from build123d import *

# Parameters (mm, degrees)
F0_W           = 15
F0_H           = 50
F1_DEPTH       = 20
F3_D           = 5.5
F3_CBORE_D     = 9.5
F3_CBORE_DEPTH = 5.4
F4_SIZE        = 1


with BuildPart() as f1:
    # F0 (on Top) → F1 (new body)
    with BuildSketch(Plane.XY):
        with Locations((7.5, 25)):
            Rectangle(F0_W, F0_H)
    extrude(amount=F1_DEPTH)

    # F3 (through all)
    with Locations(Plane.YZ.offset(15)):
        with Locations((7.5, 10), (42.5, 10)):
            CounterBoreHole(F3_D / 2, F3_CBORE_D / 2, F3_CBORE_DEPTH)

    # F4
    f4_edges = [f1.edges().sort_by_distance(p)[0] for p in [
        (15, 25, 20),
        (7.5, 0, 20),
        (0, 25, 20),
        (7.5, 50, 20),
    ]]
    chamfer(f4_edges, length=F4_SIZE)


solid = f1.part
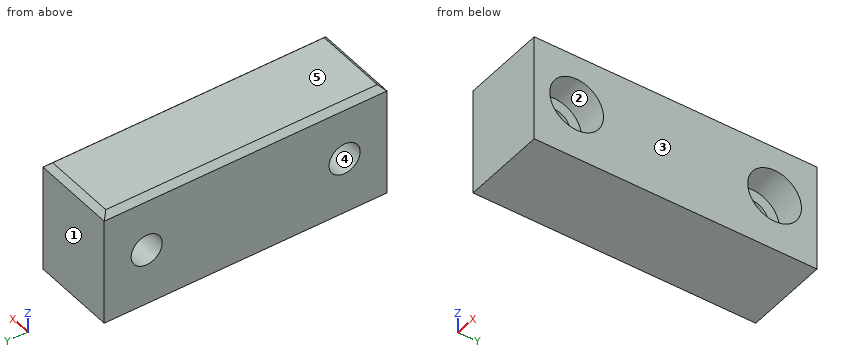
Geometry: final body of the model. Coordinates: model frame, mm. Face numbers are marked on the shaded views. A direction names the side the tool comes from. Give positions to 0.01 mm unless a question says otherwise; leave off trailing zeros. Write each loop counter-clockwise with the first axis right and the second up, starting at its lowest first coordinate (ties: lowest second). Pieces come first, ordered by that corner, then holes. Notation, with made-up numbers: M 89.25,68.25 L 114.25,68.25 A20 cw 114.25,98.25 Z; hole C 86.5,-39 d4. An arc over 180 degrees is marked long. Answer in a Markdown table with one row per item. Add a question column.
(1) Ray query, line 1 (Y direction, x = 6.5, z = 8.75); line 2 (Z direction, x = 13.6, y = 7.5); line 3 (Y direction, x = 2.25, z = 7.75). Return the intervals inside material, ascending.
(2) Mould query, pull axis Z, two halves, no side actions, for the marked faces 3, 4 and 5. Classes: +Z half, -Z half, draft (parallel to the pull), parting line (faces both ways), or undercut.
(3) Section D-D on y = 44. Return loops of the section in (x, z), and give its area (3 significant figures).
(4) Section B-B on x = 2.5. Return loops of the section in (y, z), and give its area (3 significant figures).
(5) Section A-A on z = 10. Return loops of the section in (x, y), and give its area (3 significant figures).
(6) First-contact query: pin 1 (5 mm diameter, centred on y = 8, z = 12, fed in from +X); pin 2 (4.5 mm diameter, centred on y = 42.5, z = 10, fed in from -X). Flat tips, straight axial feed; report the tip coordinate or a pass-through.
(7) Reachability of the marked faces 1 and 2 from +Z, -Z, +X, -X, +Y, -Y: full face, straight path, thin tool, end or side. Return the list, or none.
(8) Section C-C on y = 7.5. Return loops of the section in (x, z), and give its area (3 significant figures).
Result set:
| question | item | result |
|---|---|---|
| 1 | line 1 | y = 0 to 5.05, 9.95 to 40.05, 44.95 to 50 |
| 1 | line 2 | z = 0 to 5.25, 14.75 to 20 |
| 1 | line 3 | y = 0 to 5.92, 9.08 to 40.92, 44.08 to 50 |
| 2 | face 3 | draft |
| 2 | face 4 | undercut |
| 2 | face 5 | +Z half |
| 3 | outline | M 0,0 L 15,0 L 15,5.49 L 9.6,5.49 L 9.6,7.7 L 0,7.7 Z; M 0,12.3 L 9.6,12.3 L 9.6,14.51 L 15,14.51 L 15,19 L 14,20 L 1,20 L 0,19 Z |
| 3 | area | 206 mm^2 |
| 4 | outline | M 0,0 L 50,0 L 50,19 L 49,20 L 1,20 L 0,19 Z; hole C 7.5,10 d5.5; hole C 42.5,10 d5.5 |
| 4 | area | 951 mm^2 |
| 5 | outline | M 0,0 L 15,0 L 15,2.75 L 9.6,2.75 L 9.6,4.75 L 0,4.75 Z; M 0,10.25 L 9.6,10.25 L 9.6,12.25 L 15,12.25 L 15,37.75 L 9.6,37.75 L 9.6,39.75 L 0,39.75 Z; M 0,45.25 L 9.6,45.25 L 9.6,47.25 L 15,47.25 L 15,50 L 0,50 Z |
| 5 | area | 542 mm^2 |
| 6 | pin 1 | stops at x = 9.6 |
| 6 | pin 2 | passes through |
| 7 | face 1 | +Z, -Z, +X, -X, +Y |
| 7 | face 2 | +X |
| 8 | outline | M 0,0 L 15,0 L 15,5.25 L 9.6,5.25 L 9.6,7.25 L 0,7.25 Z; M 0,12.75 L 9.6,12.75 L 9.6,14.75 L 15,14.75 L 15,19 L 14,20 L 1,20 L 0,19 Z |
| 8 | area | 195 mm^2 |
